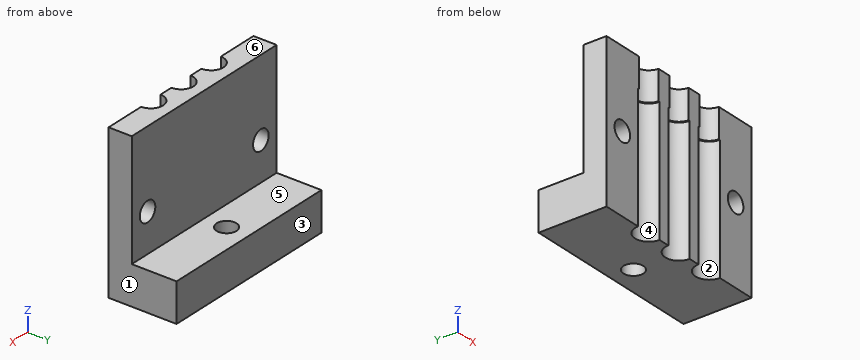
Autodesk Inventor part; units mm, degrees
ref_plane "YZ Plane" through (0, 0, 0) normal (1, 0, 0) x (0, 1, 0)
ref_plane "XZ Plane" through (0, 0, 0) normal (0, 1, 0) x (-1, 0, 0)
ref_plane "XY Plane" through (0, 0, 0) normal (0, 0, 1) x (1, 0, 0)
sketch "Sketch1" plane through (0, 0, 0) normal (0, 0, 1) x (1, 0, 0)
  circle A0 centre (-6.35, 0) radius 2.2543
  circle A1 centre (0, 0) radius 2.2543
  circle A2 centre (6.35, 0) radius 2.2543
  line L0 (-15.24, 3.81) -> (15.24, 3.81)
  line L1 (15.24, 3.81) -> (15.24, 0)
  line L2 (15.24, 0) -> (-15.24, 0)
  line L3 (-15.24, 0) -> (-15.24, 3.81)
  dimension "d0" = 4.5085
  dimension "d3" = 6.35
  dimension "d4" = 6.35
  dimension "d5" = 3.81
  dimension "d6" = 30.48
extrude "Extrusion1" add sketch "Sketch1" along normal blind 25.4 contours L2 A0 | A0 L2 L3 L0 L1 A2 A1 | A1 L2 | A2 L2 picked at (-7.1014, 0.9966) picked at (0.5625, 0.4983) picked at (6.8906, 0.6781)
extrude "Extrusion2" cut sketch "Sketch1" along normal blind 20.574 contours L2 A0 | A0 L2 | L2 A1 | A1 L2 | L2 A2 | A2 L2
sketch "Sketch2" plane through (0, 0, 25.4) normal (0, 0, 1) x (1, 0, 0)
  circle A0 centre (0, 0) radius 2.2543
  circle A1 centre (6.35, 0) radius 2.2543
  circle A2 centre (-6.35, 0) radius 2.2543
  circle A3 centre (-6.35, 0) radius 2.032
  circle A4 centre (0, 0) radius 2.032
  circle A5 centre (6.35, 0) radius 2.032
  dimension "d11" = 4.064
extrude "Extrusion3" cut sketch "Sketch2" against normal blind 4.826 contours A3 | A4 | A5
sketch "Sketch3" plane through (0, 0, 0) normal (0, 1, 0) x (-1, 0, 0)
  line L0 (15.24, 0) -> (-15.24, 0) construction
  line L1 (15.24, 0) -> (15.24, 25.4) construction
  line L2 (-15.24, 25.4) -> (15.24, 25.4) construction
  line L3 (-15.24, 0) -> (-15.24, 25.4) construction
  line L4 (-15.24, 12.7) -> (15.24, 12.7) construction
  line L5 (-8.6043, 20.574) -> (-8.6043, 0) construction
  line L6 (-11.9221, 12.7) -> (-8.6043, 12.7)
  line L7 (-11.9221, 12.7) -> (-15.24, 12.7)
hole "Hole1" at (11.9221, 0, 12.7) direction (0, 1, 0) diameter 3.2766 end through all
mirror "Mirror1" about plane through (0, 0, 0) normal (1, 0, 0) of "Hole1"
sketch "Sketch7" plane through (0, 0, 0) normal (0, 0, 1) x (1, 0, 0)
  line L0 (-15.24, 3.81) -> (15.24, 3.81)
  line L1 (15.24, 3.81) -> (-15.24, 3.81)
  line L2 (-15.24, 3.81) -> (-15.24, 11.176)
  line L3 (-15.24, 11.176) -> (15.24, 11.176)
  line L4 (15.24, 11.176) -> (15.24, 3.81)
  line L5 (-15.24, 7.493) -> (15.24, 7.493)
  point P0 (0, 7.493)
  point P1 (0, 0)
  point P2 (0, 7.493)
  dimension "d36" = 3.683
extrude "Extrusion5" add sketch "Sketch7" along normal blind 6.35
hole "Hole2" at (0, 7.493, 0) direction (0, 0, 1) diameter 3.2766 end through all
properties part number "keyhole holder"
Geometry: final body of the model. Coordinates: model frame, mm. Face numbers are marked on the shaded views. A direction names the side the tool comes from. Give positions to 0.01 mm unless a question says otherwise; leave off trailing zeros. Write each loop counter-clockwise with the first axis right and the second up, starting at its lowest first coordinate (ties: lowest second). Pieces come first, ordered by that corner, then holes. Notation, with made-up numbers: (17, 85) - (29, 85) arc R20 cw to (29, 104) - close; hole circle Ø6 at (37, -16.5). An arc over 180 degrees is marked (long way). Return JSON: item names as keys, results as strings. Group by question number.
1) First-contact query: P1, Ø2, axis at x = 2.5, y = 7.5, coming from the +Z side; P2, Ø6, axis at x = -2.5, z = 11.5, coming from the +Y side; P3, Ø6, axis at y = 7.5, z = 15, coming from the -X side (3 decimals); P4, Ø1.1, axis at x = 0.5, y = 1.5, coming from the -Z side. Flat tips, straight axial feed; report the tip coordinate or a pass-through.
2) Section C-C on z = 1.75. Return the cut outline in (x, y).
3) Section A-A on z = 12.7. Return the cut outline in (x, y), plus the area to 3 significant figures.
4) Line query: line 1 (X direction, y = 1.5, z = 23.5); line 2 (Y direction, x = 2.5, z = 19); line 3 (X direction, y = 1.45, z = 12.7). Output: solid intervals per line, ascending.
5) Section B-B on x = 0. Return the cut outline in (y, z), plus the area to 3 significant figures.
6) Set-up query: the marked faces 4, 5 and 6. Return all of +Z, -Z, +X, -X, +Y, -Y with unobstructed straight access to the full face (end or side cutting, diameter ignored); none if empty.
7) Section D-D on x = -6.35. Return the cut outline in (y, z).
8) Mould query, pull axis X, two halves, no side actions, for the marked faces 1, 2 and 3. Classes: released by +X, released by -X, zero draft, split by the parting line, or undercut.
Filled in:
{
 "1": {"P1": "stops at z = 6.35", "P2": "stops at y = 3.81", "P3": "passes through", "P4": "stops at z = 20.57"},
 "2": {"outline": "(-15.24, 0) - (-8.6, 0) arc R2.25 cw to (-4.1, 0) - (-2.25, 0) arc R2.25 cw to (2.25, 0) - (4.1, 0) arc R2.25 cw to (8.6, 0) - (15.24, 0) - (15.24, 11.18) - (-15.24, 11.18) - close; hole circle Ø3.28 at (0, 7.49)"},
 "3": {"outline": "(-15.24, 0) - (-13.56, 0) - (-13.56, 3.81) - (-15.24, 3.81) - close; (-10.28, 0) - (-8.6, 0) arc R2.25 cw to (-4.1, 0) - (-2.25, 0) arc R2.25 cw to (2.25, 0) - (4.1, 0) arc R2.25 cw to (8.6, 0) - (10.28, 0) - (10.28, 3.81) - (-10.28, 3.81) - close; (13.56, 0) - (15.24, 0) - (15.24, 3.81) - (13.56, 3.81) - close", "area": "67.2 mm^2"},
 "4": {"line 1": "x = -15.24 to -7.72, -4.98 to -1.37, 1.37 to 4.98, 7.72 to 15.24", "line 2": "y = 0 to 3.81", "line 3": "x = -15.24 to -13.56, -10.28 to -8.08, -4.62 to -1.73, 1.73 to 4.62, 8.08 to 10.28, 13.56 to 15.24"},
 "5": {"outline": "(2.03, 20.57) - (2.25, 20.57) - (2.25, 0) - (5.85, 0) - (5.85, 6.35) - (3.81, 6.35) - (3.81, 25.4) - (2.03, 25.4) - close; (9.13, 0) - (11.18, 0) - (11.18, 6.35) - (9.13, 6.35) - close", "area": "66.6 mm^2"},
 "6": {"face 4": "-Z, -Y", "face 5": "+Z, +X, -X, +Y", "face 6": "+Z, +X, -X, +Y, -Y"},
 "7": {"outline": "(2.03, 20.57) - (2.25, 20.57) - (2.25, 0) - (11.18, 0) - (11.18, 6.35) - (3.81, 6.35) - (3.81, 25.4) - (2.03, 25.4) - close"},
 "8": {"face 1": "released by +X", "face 2": "undercut", "face 3": "zero draft"}
}
